Source: CAD feature listing. Evaluate the final solid. Frame: model axes, mm. A direction names the side the tool comes from. Give positions to 0.01 mm unless a question says otherwise; leave off trailing zeros. Loops run counter-clockwise (first coordinate to the right, second up) from the corner with the lowest first, then second, coordinate; pieces in that order, holes last. Notation, with made-up numbers: M 56.25,40 L 105.25,40 A24 cw 105.25,58 Z; hole C -18,81.25 d4. An arc over 180 degrees is marked long. Answer in a Markdown table with one row per item.
```python
from build123d import *

# Parameters (mm, degrees)
SKETCH1_W           = 82.0674
SKETCH1_H           = 79.121
SKETCH1_R           = 12.7
SKETCH1_W_2         = 28.575
SKETCH1_H_2         = 58.801
BOSS_EXTRUDE1_DEPTH = 25.4
CUT_EXTRUDE1_REACH  = 118.792


with BuildPart() as part:
    # Sketch1 → Boss-Extrude1 (new body)
    with BuildSketch(Plane(origin=(0, 0, 0), x_dir=(1, 0, 0), z_dir=(0, 1, 0))):
        with Locations((-41.0337, 39.5605)):
            Rectangle(SKETCH1_W, SKETCH1_H)
        with Locations(Location((-23.495, 54.61, 0), (0, 0, 270))):
            Circle(SKETCH1_R, mode=Mode.SUBTRACT)
        with Locations((-61.4299, 39.5605)):
            Rectangle(SKETCH1_W_2, SKETCH1_H_2, mode=Mode.SUBTRACT)
    extrude(amount=BOSS_EXTRUDE1_DEPTH)

    # Sketch2 → Cut-Extrude1 (cut, up to next)
    with BuildSketch(Plane(origin=(0, 25.4, 0), x_dir=(1, 0, 0), z_dir=(0, 1, 0)), mode=Mode.PRIVATE) as cut_extrude1_sk1:
        with BuildLine():
            Line((-40.7924, 0), (-40.7924, 35.56))
            Line((-40.7924, 35.56), (-23.495, 35.56))
            ThreePointArc((-23.495, 35.56), (-4.445, 54.61), (-23.495, 73.66))
            Line((-23.495, 73.66), (-40.7924, 73.66))
            Line((-40.7924, 73.66), (-40.7924, 79.121))
            Line((-40.7924, 79.121), (0, 79.121))
            Line((0, 79.121), (0, 0))
            Line((0, 0), (-40.7924, 0))
        make_face()
    cut_extrude1_tool1 = extrude(cut_extrude1_sk1.sketch, amount=-CUT_EXTRUDE1_REACH, mode=Mode.PRIVATE) & part.part
    add(cut_extrude1_tool1.solids().sort_by_distance((-17.944529, 25.4, -30.304871))[0], mode=Mode.SUBTRACT)


solid = part.part
```
Q1. Section query A-A (z = -54.61). Output: boundary loops of the cut face in (x, y) (3 decimals).
Values follow:
| item | result |
|---|---|
| outline | M -82.067,0 L -75.717,0 L -75.717,25.4 L -82.067,25.4 Z; M -47.142,0 L -36.195,0 L -36.195,25.4 L -47.142,25.4 Z; M -10.795,0 L -4.445,0 L -4.445,25.4 L -10.795,25.4 Z |
Q2. Ray query, probe 1 along X at (y, z) = (6, -54.61) (3 decimals); probe 2 along X at (y, z) = (4.5, -19); probe 3 along Z at (x, y) = (-61.5, 22). Return the intervals inside material, ascending. Write a range as from..to.
Values follow:
| item | result |
|---|---|
| probe 1 | -82.067..-75.717, -47.142..-36.195, -10.795..-4.445 |
| probe 2 | -82.07..-75.72, -47.14..-40.79 |
| probe 3 | -79.12..-68.96, -10.16..0 |
Q3. Reachability of faces 4 (the flat face through (-40.792, 13, -18)), 5 (the flat face through (-62, 13, 0)), 6 (the flat face through (-32, 13, -73.66)), 7 (the cylindrical face through (-4.45, 12.88, -54.19)), 8 (the flat face through (-47.142, 13, -39)) from +Z, -Z, +X, -X, +Y, -Y: full face, straight path, thin tool, end or side. Return the list, or none.
Values follow:
| item | result |
|---|---|
| face 4 | +Z, +X, +Y, -Y |
| face 5 | +Z, +X, -X, +Y, -Y |
| face 6 | -Z, +X, +Y, -Y |
| face 7 | +X, +Y, -Y |
| face 8 | +Y, -Y |
Q4. Mould query, pull axis Z, two halves, no side actions, for faces 1 (the flat face through (-62, 13, -68.961)), 2 (the flat face through (-44, 0, -40)), 3 (the flat face through (-32, 13, -35.56)). Classes: +Z half, -Z half, draft (parallel to the pull), parting line (faces both ways), or undercut.
Values follow:
| item | result |
|---|---|
| face 1 | undercut |
| face 2 | draft |
| face 3 | +Z half |
Q5. Section query C-C (y = 12.25). Output: boundary loops of the cut face in (x, z) (3 decimals).
Values follow:
| item | result |
|---|---|
| outline | M -82.067,-79.121 L -40.792,-79.121 L -40.792,-73.66 L -23.495,-73.66 A19.05 ccw -23.495,-35.56 L -40.792,-35.56 L -40.792,0 L -82.067,0 Z; hole M -75.717,-68.961 L -47.142,-68.961 L -47.142,-10.16 L -75.717,-10.16 Z; hole C -23.495,-54.61 d25.4 |
Q6. Contact query for flat-ended pins moving along their axis: pin 1 Ø10 at (x, z) = (-66, -55) entering from -Y; pin 2 Ø14 at (x, y) = (-31.5, 7) entering from +Z; pin 3 Ø2.5 at (y, z) = (13, -77) entering from +X; pin 4 Ø14 at (x, y) = (-33, 14.5) entering from -Z. Output: stop coordinate, or through.
Values follow:
| item | result |
|---|---|
| pin 1 | through |
| pin 2 | z = -35.56 |
| pin 3 | x = -40.79 |
| pin 4 | z = -73.66 |
Q7. Section query B-B (x = -55). Output: boundary loops of the cut face in (y, z).
Values follow:
| item | result |
|---|---|
| outline | M 0,-79.12 L 25.4,-79.12 L 25.4,-68.96 L 0,-68.96 Z; M 0,-10.16 L 25.4,-10.16 L 25.4,0 L 0,0 Z |
Q8. Section query D-D (z = -18.5). Output: boundary loops of the cut face in (x, y), plus the area to 3 significant figures.
Values follow:
| item | result |
|---|---|
| outline | M -82.07,0 L -75.72,0 L -75.72,25.4 L -82.07,25.4 Z; M -47.14,0 L -40.79,0 L -40.79,25.4 L -47.14,25.4 Z |
| area | 323 mm^2 |
